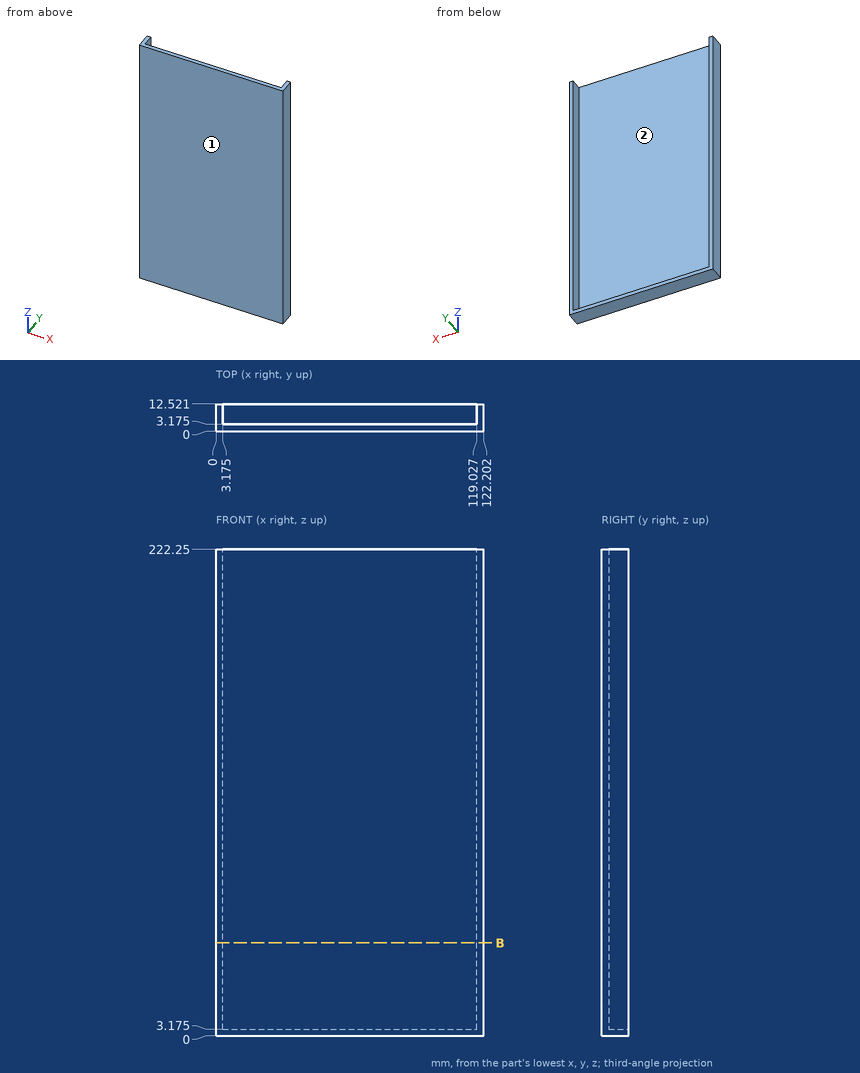
Design review of the part shown in the three views and the two pictorial views. Dimensions are in mm from the part's minimum x, y and z. A direction names the side the tool comes from. Round coordinates to 2 decimals unless told otherwise and drop trailing zeros. Loops run counter-clockwise (first coordinate to the right, second up) from the corner with the lowest first, then second, coordinate; pieces in that order, holes last. Notation, with made-up numbers: (24.25, 24) - (34.25, 24) arc R25 cw to (34.25, 62) - close; hole circle Ø11 at (61, 75). An arc over 180 degrees is marked (long way). Write each question's results on one line, items separated by ' | '. Start each with the question number.
Q1. Insertion check: P1, Ø2, axis at x = 65, y = 8.5, coming from the +Z side (3 decimals); P2, Ø1, axis at x = 39.5, z = 173, coming from the +Y side (3 decimals). Each pin has a flat end and moves straight along its axis. Give the tip position at first contact, or say it passes through.
Q2. Tool access review of the marked faces 1 and 2: name each direction out of +Z, -Z, +X, -X, +Y, -Y from which nothing blocks a thin tool from reaching the whole face with its end or side.
Q3. Wall thickness on line 1 along X through (y, z) = (9.25, 65) (1 decimal); line 2 along Z through (x, y) = (14.5, 5.5) (1 decimal): over which ranges is each line inside the solid? List them lowest first. Write a range as [from, to].
Q4. Take a section at B-B on z = 42.5. Give the boundary of the cut face in (x, y) (1 decimal).
Data:
1) P1: stops at z = 3.175 | P2: stops at y = 3.175
2) face 1: +Z, -Z, +X, -X, -Y | face 2: +Z, +Y
3) line 1: x = [0, 3.2], [119, 122.2] | line 2: z = [0, 3.2]
4) outline: (0, 0) - (122.2, 0) - (122.2, 12.5) - (119, 12.5) - (119, 3.2) - (3.2, 3.2) - (3.2, 12.5) - (0, 12.5) - close
